Verification items for the finished model (mm, model axes). Round coordinates to 2 decimals unless told otherwise and drop trailing zeros. Order: outer loops, then holes, each group sorted by start corner. A loop starts at its lowest first (then second) coordinate and runs counter-clockwise, first axis right, second up. Notation, with made-up numbers: (62.25, 5) -> (74.25, 5) arc R12 ccw to (74.25, 18) -> close; hole circle Ø8 at (-10.75, 49). An arc over 180 degrees is marked (long way). Return JSON: item names as keys, results as strings. Group by question number.
1) Section check A-A on z = 90. Enter the section's corners in (x, y).
2) Section check D-D on z = -538.5. Enter the section's corners in (x, y), plus the area to 3 significant figures.
3) Section check C-C on y = 742.5. Enter the section's corners in (x, z), plus the area to 3 significant figures.
4) Section check B-B on x = 11.75. Enter the section's corners in (y, z), plus the area to 3 significant figures.
5) Depth check by flat-ended pin: pin 1 (12 mm diameter, centred on x = 16.5, y = -104, fed in from -Z); pin 2 (5 mm diameter, centred on x = 15, y = -171, fed in from -Z); pin 3 (6 mm diameter, centred on x = 11.5, y = 716.5, fed in from +Z). Enter the tip coordinate at first touch or a pass-through.
6) Scan lines: L1, parallel to Z at x = 12.5, y = 789.5; L2, parallel to Y at x = 11.75, z = -535; L3, parallel to Y at x = 7.75, z = 65. Record each from-to range of solid material in increasing order.
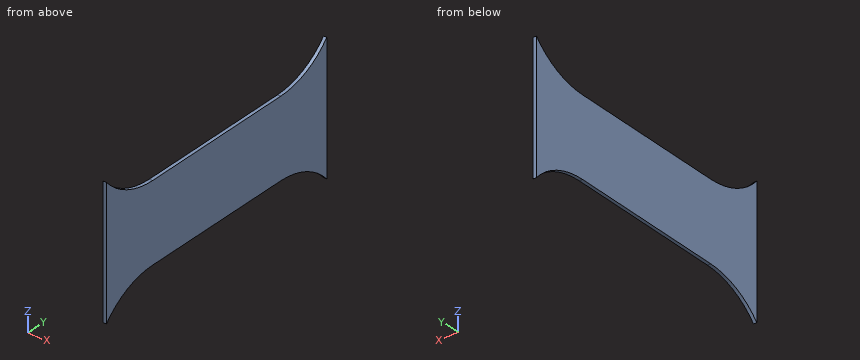
```python
from build123d import *

# Parameters (mm, degrees)
BOSS_EXTRUDE1_DEPTH = 20
CUT_EXTRUDE1_DEPTH  = 20


with BuildPart() as part:
    # Sketch1 → Boss-Extrude1 (new body)
    with BuildSketch(Plane(origin=(0, 0, 0), x_dir=(0, 0, -1), z_dir=(1, 0, 0))):
        with BuildLine():
            Line((0, 0), (0, 972))
            ThreePointArc((0, 972), (-134.730880654, 1297.269119346), (-460, 1432))
            Line((-460, 1432), (940, 1432))
            ThreePointArc((940, 1432), (614.730880654, 1297.269119346), (480, 972))
            Line((480, 972), (480, 0))
            ThreePointArc((480, 0), (614.730880654, -325.269119346), (940, -460))
            Line((940, -460), (-460, -460))
            ThreePointArc((-460, -460), (-134.730880654, -325.269119346), (0, 0))
        make_face()
    extrude(amount=BOSS_EXTRUDE1_DEPTH)

    # Sketch2 → Cut-Extrude1 (cut)
    with BuildSketch(Plane(origin=(20, 0, 0), x_dir=(0, 0, -1), z_dir=(1, 0, 0))):
        Polygon((-460, 1322), (1004.695967819, 1322), (1004.695967819, 1530.227687148), (-489.352876869, 1530.227687148), align=None)
        Polygon((1004.695967819, -350), (1004.695967819, -558.227687148), (-489.352876869, -558.227687148), (-460, -350), align=None)
    extrude(amount=-CUT_EXTRUDE1_DEPTH, mode=Mode.SUBTRACT)


solid = part.part
```
Check result:
{
 "1": {"outline": "(0, -350) -> (20, -350) -> (20, -273.31) -> (0, -273.31) -> close; (0, 1245.31) -> (20, 1245.31) -> (20, 1322) -> (0, 1322) -> close"},
 "2": {"outline": "(0, -350) -> (20, -350) -> (20, -224.49) -> (0, -224.49) -> close; (0, 1196.49) -> (20, 1196.49) -> (20, 1322) -> (0, 1322) -> close", "area": "5,020 mm^2"},
 "3": {"outline": "(0, -480) -> (20, -480) -> (20, 0) -> (0, 0) -> close", "area": "9,600 mm^2"},
 "4": {"outline": "(-350, -641.5) arc R460 cw to (0, -480) -> (972, -480) arc R460 cw to (1322, -641.5) -> (1322, 161.5) arc R460 cw to (972, 0) -> (0, 0) arc R460 cw to (-350, 161.5) -> close", "area": "872,000 mm^2"},
 "5": {"pin 1": "z = -493.35", "pin 2": "z = -513.97", "pin 3": "z = 0"},
 "6": {"L1": "-480 to 0", "L2": "-350 to -218.12, 1190.12 to 1322", "L3": "-350 to -235.74, 1207.74 to 1322"}
}
